from build123d import *

# Parameters (mm, degrees)
SKETCH1_W                             = 127
SKETCH1_H                             = 114.3
BOSS_EXTRUDE1_DEPTH                   = 9.525
SKETCH2_R                             = 12.7
CUT_EXTRUDE1_DEPTH                    = 86.959863454
F_10_CLEARANCE_HOLE2_D                = 5.1054
F_10_CLEARANCE_HOLE2_DEPTH            = 38.1
F_10_CLEARANCE_HOLE2_TIP              = 1.533816902
F_10_CLEARANCE_HOLE3_D                = 5.1054
TAPPED_HOLE_FOR_10_32_HELICOIL1_D     = 5.1054
TAPPED_HOLE_FOR_10_32_HELICOIL1_DEPTH = 25.4
TAPPED_HOLE_FOR_10_32_HELICOIL1_TIP   = 1.533816902
CHAMFER1_SIZE                         = 0.508


with BuildPart() as part:
    # Sketch1 → Boss-Extrude1 (new body)
    with BuildSketch(Plane(origin=(0, 0, 0), x_dir=(1, 0, 0), z_dir=(0, 1, 0))):
        Rectangle(SKETCH1_W, SKETCH1_H)
    extrude(amount=BOSS_EXTRUDE1_DEPTH)

    # Sketch2 → Cut-Extrude1 (cut, through all)
    with BuildSketch(Plane(origin=(0, 9.525, 0), x_dir=(1, 0, 0), z_dir=(0, 1, 0))):
        with Locations(Location((-3.4925, -1.5494, 0), (0, 0, 270))):
            Circle(SKETCH2_R)
    extrude(amount=-CUT_EXTRUDE1_DEPTH, mode=Mode.SUBTRACT)

    # #10 Clearance Hole2
    with Locations(Plane(origin=(1.014314116, 0, 37.659468055), x_dir=(1, 0, 0), z_dir=(0, -1, 0))):
        with Locations((-35.395754116, -74.210068055), (33.184245884, 1.989931945), (-35.395754116, 1.989931945), (33.184245884, -74.210068055)):
            Hole(F_10_CLEARANCE_HOLE2_D / 2, depth=F_10_CLEARANCE_HOLE2_DEPTH)
            with Locations((0, 0, -(F_10_CLEARANCE_HOLE2_DEPTH + F_10_CLEARANCE_HOLE2_TIP / 2))):  # 118° drill point
                Cone(0, F_10_CLEARANCE_HOLE2_D / 2, F_10_CLEARANCE_HOLE2_TIP, mode=Mode.SUBTRACT)

    # #10 Clearance Hole3 (through all)
    with Locations(Plane(origin=(0, 0, 0), x_dir=(-1, 0, 0), z_dir=(0, -1, 0))):
        with Locations((-54.0385, 33.02), (-57.0865, -8.128), (57.0865, 33.02), (54.0385, -8.128)):
            Hole(F_10_CLEARANCE_HOLE3_D / 2)

    # Tapped Hole for #10-32 Helicoil1
    with Locations(Plane.XY.offset(57.15)):
        with Locations((-53.18125, 4.7625), (15.08125, 4.7625)):
            Hole(TAPPED_HOLE_FOR_10_32_HELICOIL1_D / 2, depth=TAPPED_HOLE_FOR_10_32_HELICOIL1_DEPTH)
            with Locations((0, 0, -(TAPPED_HOLE_FOR_10_32_HELICOIL1_DEPTH + TAPPED_HOLE_FOR_10_32_HELICOIL1_TIP / 2))):  # 118° drill point
                Cone(0, TAPPED_HOLE_FOR_10_32_HELICOIL1_D / 2, TAPPED_HOLE_FOR_10_32_HELICOIL1_TIP, mode=Mode.SUBTRACT)

    # Chamfer1
    chamfer1_edges = [part.edges().sort_by_distance(p)[0] for p in [
        (-63.5, 9.525, 0),
        (0, 9.525, 57.15),
        (-3.4925, 0, -11.1506),
        (-3.4925, 9.525, -11.1506),
        (36.75126, 9.525, -36.5506),
        (36.75126, 0, -36.5506),
        (-31.82874, 9.525, 39.6494),
        (-31.82874, 0, 39.6494),
        (36.75126, 9.525, 39.6494),
        (36.75126, 0, 39.6494),
        (-31.82874, 9.525, -36.5506),
        (-31.82874, 0, -36.5506),
        (63.5, 9.525, 0),
        (-56.5912, 0, 8.128),
        (-56.5912, 9.525, 8.128),
        (0, 0, 57.15),
        (-59.6392, 0, -33.02),
        (-59.6392, 9.525, -33.02),
        (-63.5, 0, 0),
        (0, 0, -57.15),
        (54.5338, 0, 8.128),
        (54.5338, 9.525, 8.128),
        (63.5, 0, 0),
        (51.4858, 0, -33.02),
        (51.4858, 9.525, -33.02),
        (17.63395, 4.7625, 57.15),
        (-50.62855, 4.7625, 57.15),
        (0, 9.525, -57.15),
        (63.5, 4.7625, 57.15),
        (-63.5, 4.7625, 57.15),
        (-63.5, 4.7625, -57.15),
        (63.5, 4.7625, -57.15),
    ]]
    chamfer(chamfer1_edges, length=CHAMFER1_SIZE)


solid = part.part
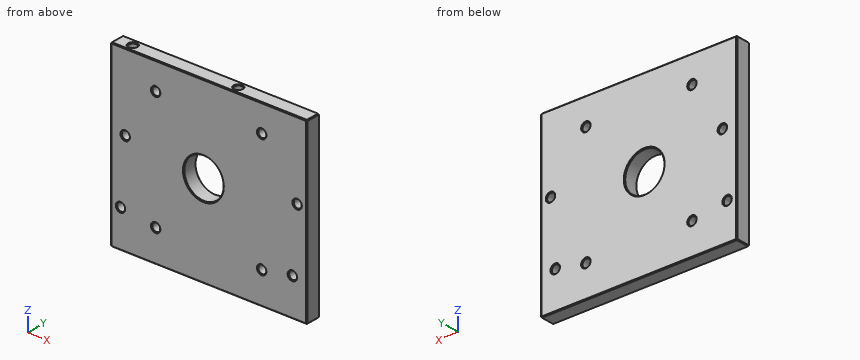
Read the model definition and answer for the solid it produces. Units are mm, in the model's axes. Coordinates: 2 decimals unless noted, no trailing zeros. Order: outer loops, then holes, each group sorted by start corner. A loop starts at its lowest first (then second) coordinate and runs counter-clockwise, first axis right, second up. Notation, with made-up numbers: (-1.75, 21.25) -> (39.25, 21.25) arc R34 cw to (39.25, 59.25) -> close; hole circle Ø10 at (64.5, 84.25). An arc over 180 degrees is marked (long way). Answer as a JSON object with one key per item and string values.
1) This flat-tipped pin is pushed along its axis until it touches: pin 1 (4.5 mm diameter, centred on x = 15.08, y = 4.76, fed in from +Z). Where does it stop, or does it pass through?
Model answer:
{"pin 1": "stops at z = 31.57"}
2) Consider line 1 along Z through (x, y) = (-34.5, 4); line 2 along X through (y, z) = (7.25, -33.02); line 3 along Z through (x, y) = (-33, 8). Determine where each line is inside the solid, lowest interval first. Write a range as from..to.
Model answer:
{"line 1": "z = -57.15..-39.1, -34..37.1, 42.2..57.15", "line 2": "x = -63.5..-59.64, -54.53..51.49, 56.59..63.5", "line 3": "z = -57.15..-38.7, -34.4..37.5, 41.8..57.15"}
3) A cutting plane is placed at A-A, the plane z = 45. Determine the outline of the cut face in (x, y) (1 decimal), plus the area to 3 significant figures.
Model answer:
{"outline": "(-63.5, 0.5) -> (-63, 0) -> (63, 0) -> (63.5, 0.5) -> (63.5, 9) -> (63, 9.5) -> (-63, 9.5) -> (-63.5, 9) -> close; hole circle Ø5.1 at (-53.2, 4.8); hole circle Ø5.1 at (15.1, 4.8)", "area": "1,170 mm²"}
